Source: CAD feature listing. Evaluate the final solid. Frame: model axes, mm. Give positions to 0.01 mm unless a question says otherwise; leave off trailing zeros. Loops run counter-clockwise (first coordinate to the right, second up) from the corner with the lowest first, then second, coordinate; pieces in that order, holes last. Notation, with made-up numbers: (38, -7.75) -> (69, -7.75) arc R10 cw to (69, 8.25) -> close; hole circle Ø5 at (79, -30). An arc over 180 degrees is marked (long way). Return JSON: item names as keys, results as strings. Group by question number.
(1) Draft query along Y for faces 1 (the face through (75, -87, 5)), 2 (the face through (71.094, -81.476, 2.465)), 3 (the face through (70.96, -89.02, 2.46)), 4 (the face through (76.76, -94.63, 2.46)). Return one class per face: released by +Y, released by -Y, zero draft, split by the parting line, or undercut.
(2) Ray query, line 1 (Y direction, x = 74, z = 2.4); line 2 (Y direction, x = 71.75, z = 3.6); line 3 (X direction, y = -80, z = 4.8). Return the intervals inside material, ascending. Write a range as from..to.
(3) Cut plane A-A on x = 74. Return loops of the section in (y, z).
(4) Cut plane D-D on x = 82.75. Return loops of the section in (y, z), then the cut area to 3 significant figures.
(5) Cut plane B-B on y = -80.5. Return loops of the section in (x, z), then the cut area to 3 significant figures.
Autodesk Inventor part; units mm, degrees
ref_plane "YZ Plane" through (0, 0, 0) normal (1, 0, 0) x (0, 1, 0)
ref_plane "XZ Plane" through (0, 0, 0) normal (0, 1, 0) x (-1, 0, 0)
ref_plane "XY Plane" through (0, 0, 0) normal (0, 0, 1) x (1, 0, 0)
sketch "Sketch3" plane through (0, 0, 0) normal (0, 0, 1) x (1, 0, 0)
  line L0 (71.8451, -79.0914) -> (79.2409, -94.9518) construction
  line L1 (67.3136, -81.2045) -> (74.7094, -97.0649)
  line L2 (83.7725, -92.8387) -> (76.3766, -76.9783)
  arc A0 (76.3766, -76.9783) -> (67.3136, -81.2045) centre (71.8451, -79.0914) ccw
  arc A1 (74.7094, -97.0649) -> (83.7725, -92.8387) centre (79.2409, -94.9518) ccw
  line L3 (79.2409, -94.9518) -> (71.8451, -79.0914)
  point P0 (0, 0)
  point P1 (75.543, -87.0216)
  dimension "d16" = 10
extrude "Extrusion2" add sketch "Sketch3" along normal blind 5
sketch "Sketch4" plane through (0, 0, 5) normal (0, 0, 1) x (1, 0, 0)
  line L0 (67.3136, -81.2045) -> (74.7094, -97.0649)
  arc A0 (74.7094, -97.0649) -> (83.7725, -92.8387) centre (79.2409, -94.9518) ccw
  line L1 (83.7725, -92.8387) -> (76.3766, -76.9783)
  arc A1 (76.3766, -76.9783) -> (67.3136, -81.2045) centre (71.8451, -79.0914) ccw
  point P0 (0, 0)
hole "Hole1" at (71.8451, -79.0914, 5) at (79.2409, -94.9518, 5) direction (0, 0, -1) diameter 5 end through all
properties part number "avstandsstykke"
Answers:
{
 "1": {"face 1": "zero draft", "face 2": "undercut", "face 3": "released by -Y", "face 4": "undercut"},
 "2": {"line 1": "-95.54..-80.36, -77.82..-74.58", "line 2": "-90.72..-81.59, -76.59..-74.09", "line 3": "66.93..69.52, 74.17..77.79"},
 "3": {"outline": "(-95.54, 0) -> (-80.36, 0) -> (-80.36, 5) -> (-95.54, 5) -> close; (-77.82, 0) -> (-74.58, 0) -> (-74.58, 5) -> (-77.82, 5) -> close"},
 "4": {"outline": "(-98.51, 0) -> (-90.65, 0) -> (-90.65, 5) -> (-98.51, 5) -> close", "area": "39.3 mm²"},
 "5": {"outline": "(67.05, 0) -> (69.78, 0) -> (69.78, 5) -> (67.05, 5) -> close; (73.91, 0) -> (78.02, 0) -> (78.02, 5) -> (73.91, 5) -> close", "area": "34.2 mm²"}
}
